Autodesk Inventor part; units mm, degrees
ref_plane "YZ Plane" through (0, 0, 0) normal (1, 0, 0) x (0, 1, 0)
ref_plane "XZ Plane" through (0, 0, 0) normal (0, 1, 0) x (-1, 0, 0)
ref_plane "XY Plane" through (0, 0, 0) normal (0, 0, 1) x (1, 0, 0)
sketch "Sketch1" plane through (0, 0, 0) normal (0, 0, 1) x (1, 0, 0)
  line L0 (0, 0) -> (0, 7.62)
  line L1 (0, 0) -> (6.35, 0)
  line L2 (0, 7.62) -> (73.3235, 7.62) construction
  line L3 (6.35, 0) -> (6.35, 7.62)
  line L4 (6.35, 7.62) -> (13.3564, 7.62) construction
  line L5 (0, 7.62) -> (71.842, 79.462)
  line L6 (6.35, 7.62) -> (75.017, 76.287)
  arc A0 (75.017, 76.287) -> (71.842, 79.462) centre (73.4295, 77.8745) ccw
  dimension "d0" = 7.62
  dimension "d1" = 6.35
  dimension "d8" = 7.62
  dimension "d27" = 101.6
  dimension "d28" = 45
extrude "Extrusion4" add sketch "Sketch1" along normal blind 6.35
properties part number "Funneling_v1"
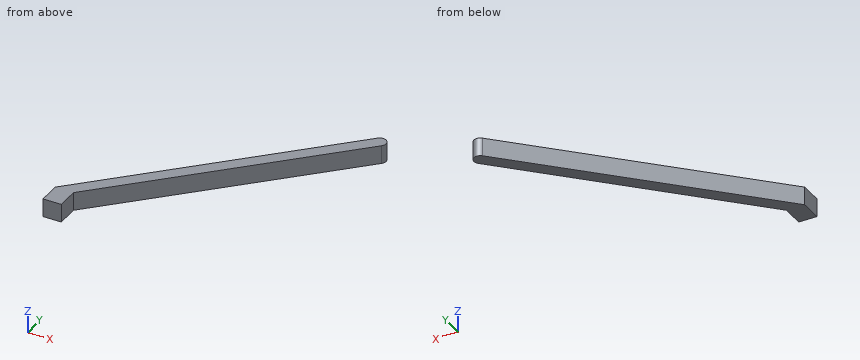
Geometry: final body of the model. Coordinates: model frame, mm. Coordinates: 2 decimals unless noted, no trailing zeros. Order: outer loops, then holes, each group sorted by start corner. A loop starts at its lowest first (then second) coordinate and runs counter-clockwise, first axis right, second up. Notation, with made-up numbers: (-25.5, 71.25) - (28.5, 71.25) arc R17 ccw to (28.5, 92.25) - close; hole circle Ø3 at (39.5, 32). An arc over 180 degrees is marked (long way). Return JSON: item names as keys, results as strings. Group by question number.
1. Cut plane C-C (y = 49). Output: boundary loops of the cut face in (x, z).
2. Material intervals for line 1 along X through (y, z) = (4.5, 5.75); line 2 along X through (y, z) = (34.5, 6.25); line 3 along Y through (x, z) = (23.5, 3.75), sorted ascending. Write a range as [from, to].
3. Pin query (flat end, axial travel): pin 1 (1.5 mm diameter, centred on x = 43.5, z = 3, fed in from +Y); pin 2 (3 mm diameter, centred on y = 24.5, z = 3.5, fed in from -X); pin 3 (1.5 mm diameter, centred on x = 43, z = 4, fed in from +Y). Return the tip coordinate at first contact, or that it passes through.
4. Cut plane A-A (z = 2). Output: boundary loops of the cut face in (x, y).
5. Cut plane B-B (x = 49). Output: boundary loops of the cut face in (y, z).
Resolved:
{
 "1": {"outline": "(41.38, 0) - (47.73, 0) - (47.73, 6.35) - (41.38, 6.35) - close"},
 "2": {"line 1": "x = [0, 6.35]", "line 2": "x = [26.88, 33.23]", "line 3": "y = [24.77, 31.12]"},
 "3": {"pin 1": "stops at y = 51.87", "pin 2": "stops at x = 15.38", "pin 3": "stops at y = 51.37"},
 "4": {"outline": "(0, 0) - (6.35, 0) - (6.35, 7.62) - (75.02, 76.29) arc R2.25 ccw to (71.84, 79.46) - (0, 7.62) - close"},
 "5": {"outline": "(50.27, 0) - (56.62, 0) - (56.62, 6.35) - (50.27, 6.35) - close"}
}
